```python
from build123d import *

# Parameters (mm, degrees)
SKETCH2_W           = 26.6
SKETCH2_H           = 36.9
SKETCH2_W_2         = 22.6
SKETCH2_H_2         = 8.3
BOSS_EXTRUDE2_DEPTH = 35
FILLET1_R           = 1
CHAMFER1_SIZE       = 0.5
CUT_EXTRUDE1_REACH  = 54.569
SKETCH3_R           = 1.5


with BuildPart() as part:
    # Sketch2 → Boss-Extrude2 (new body)
    with BuildSketch(Plane(origin=(0, 0, 0), x_dir=(1, 0, 0), z_dir=(0, 1, 0))):
        with Locations((0, -2)):
            Rectangle(SKETCH2_W, SKETCH2_H)
        with Locations((0, -10.3)):
            Rectangle(SKETCH2_W_2, SKETCH2_H_2, mode=Mode.SUBTRACT)
        Rectangle(SKETCH2_W_2, SKETCH2_H_2, mode=Mode.SUBTRACT)
        with Locations((0, 10.3)):
            Rectangle(SKETCH2_W_2, SKETCH2_H_2, mode=Mode.SUBTRACT)
    extrude(amount=BOSS_EXTRUDE2_DEPTH)

    # Fillet1
    fillet1_edges = [part.edges().sort_by_distance(p)[0] for p in [
        (-11.3, 17.5, 6.15),
        (-11.3, 17.5, 14.45),
        (11.3, 17.5, 14.45),
        (11.3, 17.5, 6.15),
        (-11.3, 17.5, -4.15),
        (-11.3, 17.5, 4.15),
        (11.3, 17.5, 4.15),
        (11.3, 17.5, -4.15),
        (-11.3, 17.5, -14.45),
        (-11.3, 17.5, -6.15),
        (11.3, 17.5, -6.15),
        (11.3, 17.5, -14.45),
    ]]
    fillet(fillet1_edges, radius=FILLET1_R)

    # Chamfer1
    chamfer1_edges = [part.edges().sort_by_distance(p)[0] for p in [
        (13.3, 35, 2),
        (0, 35, -16.45),
        (-13.3, 35, 2),
        (0, 0, -16.45),
        (13.3, 0, 2),
        (0, 0, 20.45),
        (0, 0, 14.45),
        (0, 35, 14.45),
        (11.3, 0, 10.3),
        (-13.3, 0, 2),
        (11.3, 35, 10.3),
        (-11.3, 0, 10.3),
        (-11.3, 35, 10.3),
        (0, 0, 6.15),
        (0, 35, 6.15),
        (0, 0, 4.15),
        (0, 35, 4.15),
        (11.3, 0, 0),
        (11.3, 35, 0),
        (0, 0, -4.15),
        (0, 35, -4.15),
        (-11.3, 0, 0),
        (-11.3, 35, 0),
        (11.3, 0, -10.3),
        (-13.3, 17.5, -16.45),
        (11.3, 35, -10.3),
        (13.3, 17.5, -16.45),
        (13.3, 17.5, 20.45),
        (0, 0, -14.45),
        (0, 35, -14.45),
        (-13.3, 17.5, 20.45),
        (0, 0, -6.15),
        (0, 35, -6.15),
        (-11.3, 0, -10.3),
        (-11.3, 35, -10.3),
        (11.007106781, 0, 14.157106781),
        (11.007106781, 35, 14.157106781),
        (-11.007106781, 0, 14.157106781),
        (-11.007106781, 35, 14.157106781),
        (0, 35, 20.45),
        (-11.007106781, 0, 6.442893219),
        (-11.007106781, 35, 6.442893219),
        (11.007106781, 0, 6.442893219),
        (11.007106781, 35, 6.442893219),
        (11.007106781, 0, 3.857106781),
        (11.007106781, 35, 3.857106781),
        (11.007106781, 0, -3.857106781),
        (11.007106781, 35, -3.857106781),
        (-11.007106781, 0, -3.857106781),
        (-11.007106781, 35, -3.857106781),
        (-11.007106781, 0, 3.857106781),
        (-11.007106781, 35, 3.857106781),
        (11.007106781, 0, -14.157106781),
        (11.007106781, 35, -14.157106781),
        (11.007106781, 0, -6.442893219),
        (11.007106781, 35, -6.442893219),
        (-11.007106781, 0, -14.157106781),
        (-11.007106781, 35, -14.157106781),
        (-11.007106781, 0, -6.442893219),
        (-11.007106781, 35, -6.442893219),
    ]]
    chamfer(chamfer1_edges, length=CHAMFER1_SIZE)

    # Sketch3 → Cut-Extrude1 (cut, up to next)
    with BuildSketch(Plane.XY.offset(20.45), mode=Mode.PRIVATE) as cut_extrude1_sk1:
        with Locations((0, 29)):
            Circle(SKETCH3_R)
    cut_extrude1_tool1 = extrude(cut_extrude1_sk1.sketch, amount=-CUT_EXTRUDE1_REACH, mode=Mode.PRIVATE) & part.part
    # Sketch3 → Cut-Extrude1 (cut, up to next)
    with BuildSketch(Plane.XY.offset(20.45), mode=Mode.PRIVATE) as cut_extrude1_sk2:
        with Locations((0, 6)):
            Circle(SKETCH3_R)
    cut_extrude1_tool2 = extrude(cut_extrude1_sk2.sketch, amount=-CUT_EXTRUDE1_REACH, mode=Mode.PRIVATE) & part.part
    add(cut_extrude1_tool1.solids().sort_by_distance((0, 29, 20.45))[0], mode=Mode.SUBTRACT)
    add(cut_extrude1_tool2.solids().sort_by_distance((0, 6, 20.45))[0], mode=Mode.SUBTRACT)


solid = part.part
```
Here's how the part is built. I have some questions about the finished solid (model axes, mm). A direction names the side the tool comes from. Coordinates: 2 decimals unless noted, no trailing zeros. Order: outer loops, then holes, each group sorted by start corner. A loop starts at its lowest first (then second) coordinate and runs counter-clockwise, first axis right, second up. Notation, with made-up numbers: (88.5, 70.25) - (110.5, 70.25) arc R23 cw to (110.5, 83.25) - close; hole circle Ø4 at (75.25, 53). An arc over 180 degrees is marked (long way). One line per question, with ' | ' between items. Start each with the question number.
1. I'm going to push flat-ended pins straight in: pin 1 Ø1.8 at (x, y) = (0, 6) entering from +Z; pin 2 Ø4 at (x, z) = (-7.5, 8) entering from -Y. Where does each tip first touch, or does it pass through?
2. Please list where these lines run through material, in increasing order: line 1 along Z through (x, y) = (-10, 17); line 2 along X through (y, z) = (8.5, 7). Write a range as [from, to].
3. If we mould it in two halves opening along Z, with no side actions, what happens to faces 1 (the flat face through (0, 17, -16.45)), 2 (the flat face through (-13.3, 17, 2)), 3 (the cylindrical face through (10.999, 17.738, 3.865)), 4 (the conical face through (-11.15, 34.69, -6.32))? For each: released by +Z, released by -Z, zero draft, split by the parting line, or undercut.
4. Which directions (+Z, -Z, +X, -X, +Y, -Y) give clear straight access to the entire face, cutting with the end or side of a thin tool? Please do faces 5 (the flat face through (0, 17, 6.15)), 6 (the conical face through (11.13, 34.69, -6.3)), 7 (the conical face through (11.14, 0.3, 14.31)).
5. If we section it at B-B (z = 8.5): Write out the boundary of the cut face in (x, y), and give its area (3 significant figures).
6. If we section it at A-A (x = 7.5): Give the number of separate pieces and of enclosed holes in the cut face, and give its area (3 significant figures).
Model answer:
1) pin 1: stops at z = 6.15 | pin 2: stops at y = 0.35
2) line 1: z = [-16.45, -14.45], [-6.15, -4.15], [4.15, 6.15], [14.45, 20.45] | line 2: x = [-13.3, -11.29], [11.29, 13.3]
3) face 1: released by -Z | face 2: zero draft | face 3: undercut | face 4: undercut
4) face 5: +Y, -Y | face 6: +Y | face 7: -Y
5) outline: (-13.3, 0.5) - (-12.8, 0) - (-11.8, 0) - (-11.3, 0.5) - (-11.3, 34.5) - (-11.8, 35) - (-12.8, 35) - (-13.3, 34.5) - close; (11.3, 0.5) - (11.8, 0) - (12.8, 0) - (13.3, 0.5) - (13.3, 34.5) - (12.8, 35) - (11.8, 35) - (11.3, 34.5) - close | area: 139 mm²
6) separate pieces: 4 | enclosed holes: 0 | area: 418 mm²
